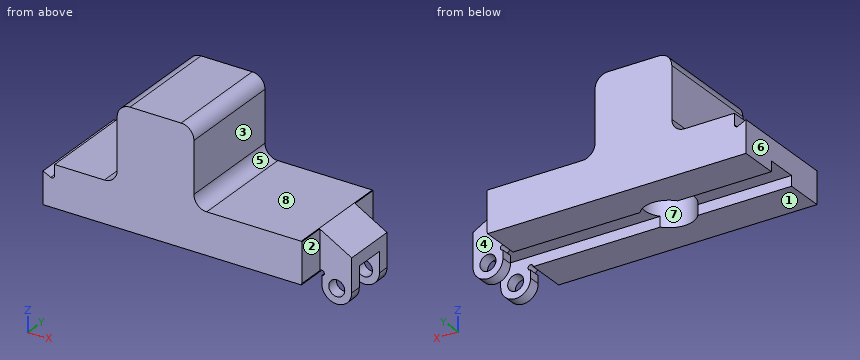
from build123d import *

# Parameters (mm, degrees)
F0_R     = 0.79375
F1_DEPTH = 10.7442
F2_W     = 2.7051
F2_H     = 1.8288
F2_H_2   = 3.302
F2_H_3   = 1.4859
F3_DEPTH = 3.175
F4_R     = 2.413
F5_DEPTH = 11.43
F6_R     = 1.27
F7_R     = 0.254
F8_W     = 3.048
F8_H     = 2.032
F8_H_2   = 1.4859
F9_DEPTH = 28.8808


with BuildPart() as f1:
    # F0 (on Front) → F1 (new body)
    with BuildSketch(Plane.XZ):
        with BuildLine():
            Line((-11.176, 3.175), (-11.176, 0))
            Line((-11.176, 0), (14.478, 0))
            ThreePointArc((14.478, 0), (14.9116051224, 0.1796051224), (14.732, -0.254))
            Line((14.732, -0.254), (14.732, -1.016))
            ThreePointArc((14.732, -1.016), (16.2179, -2.5019), (17.7038, -1.016))
            Line((17.7038, -1.016), (17.7038, 2.286))
            Line((17.7038, 2.286), (14.4678382203, 4.1148))
            Line((14.4678382203, 4.1148), (3.81, 4.1148))
            Line((3.81, 4.1148), (3.81, 11.7348))
            Line((3.81, 11.7348), (-3.81, 11.7348))
            Line((-3.81, 11.7348), (-3.81, 4.1148))
            Line((-3.81, 4.1148), (-10.033, 4.1148))
            Line((-10.033, 4.1148), (-10.033, 2.6214198342))
            Line((-10.033, 2.6214198342), (-11.176, 3.175))
        make_face()
        with Locations((16.2179, -1.016)):
            Circle(F0_R, mode=Mode.SUBTRACT)
    extrude(amount=F1_DEPTH)

    # F2 (on face) → F3 (cut)
    with BuildSketch(Plane.YZ.offset(17.7038)):
        with Locations((-9.39165, 3.2004)):
            Rectangle(F2_W, F2_H)
        with Locations((-9.39165, 0.635)):
            Rectangle(F2_W, F2_H_2)
        with Locations((-9.39165, -1.75895)):
            Rectangle(F2_W, F2_H_3)
        with Locations((-1.35255, 3.2004)):
            Rectangle(F2_W, F2_H)
        with Locations((-1.35255, 0.635)):
            Rectangle(F2_W, F2_H_2)
        with Locations((-1.35255, -1.75895)):
            Rectangle(F2_W, F2_H_3)
    extrude(amount=-F3_DEPTH, mode=Mode.SUBTRACT)

    # F4 (on face) → F5 (cut)
    with BuildSketch(Plane(origin=(0, 0, 0), x_dir=(1, 0, 0), z_dir=(0, 0, -1))):
        with Locations((0, 5.3721)):
            Circle(F4_R)
    extrude(amount=-F5_DEPTH, mode=Mode.SUBTRACT)

    # F6
    f6_edges = [f1.edges().sort_by_distance(p)[0] for p in [
        (-3.81, -5.3721, 4.1148),
        (3.81, -5.3721, 4.1148),
        (-3.81, -5.3721, 11.7348),
        (3.81, -5.3721, 11.7348),
    ]]
    fillet(f6_edges, radius=F6_R)

    # F7
    f7_edges = [f1.edges().sort_by_distance(p)[0] for p in [
        (-10.033, -5.3721, 2.62142),
    ]]
    fillet(f7_edges, radius=F7_R)

    # F8 (on face) → F9 (cut, through all)
    with BuildSketch(Plane.YZ.offset(17.7038)):
        with Locations((-5.3721, 0)):
            Rectangle(F8_W, F8_H)
        with Locations((-5.3721, -1.75895)):
            Rectangle(F8_W, F8_H_2)
    extrude(amount=-F9_DEPTH, mode=Mode.SUBTRACT)


solid = f1.part
Source: CAD feature listing. Evaluate the final solid. Frame: model axes, mm. Face numbers are marked on the shaded views. A direction names the side the tool comes from. Round coordinates to 2 decimals unless told otherwise and drop trailing zeros. Write each loop counter-clockwise with the first axis right and the second up, starting at its lowest first coordinate (ties: lowest second). Pieces come first, ordered by that corner, then holes. Notation, with made-up numbers: M -34.5,85 L 7.5,85 A25 ccw 7.5,110 Z; hole C -10.75,58 d10. An arc over 180 degrees is marked long. One line per item, written item: value. Start each with the question number.
Item 1: Mould query, pull axis X, two halves, no side actions, for the marked faces 5, 6, 7 and 8. Classes: pulls with the +X half, pulls with the -X half, needs draft (parallel to the pull), parting line crosses it, or undercut.
Item 2: Pin query (flat end, axial travel): pin 1 (1.4 mm diameter, centred on x = 16.22, z = -1.02, fed in from -Y); pin 2 (0.8 mm diameter, centred on y = -7.5, z = -0.5, fed in from -X); pin 3 (1.4 mm diameter, centred on y = -1.5, z = 3, fed in from +X); pin 4 (1.5 mm diameter, centred on x = -3, y = -1.5, fed in from -Z). Return the tip coordinate at first contact, or that it passes through.
Item 3: Set-up query: the marked faces 1, 2, 3 and 4. Return all of +Z, -Z, +X, -X, +Y, -Y with unobstructed straight access to the full face (end or side cutting, diameter ignored); none if empty.
Item 4: Ray query, L1, parallel to Z at x = 13.25, y = -2.25; L2, parallel to Y at x = -4, z = 0.75; L3, parallel to Z at x = 2.5, y = -8.5. Return the intervals inside material, ascending. Write a range as from..to.
Item 5: Section query C-C (z = 7). Return the cut outline in (x, y), plus the area to 3 significant figures.
Item 6: Section query A-A (x = 6.5). Return the cut outline in (y, z), plus the area to 3 significant figures.
Item 7: Section query B-B (y = -10). Return the cut outline in (x, z) (3 decimals).
Result set:
1. face 5: pulls with the +X half
1. face 6: pulls with the -X half
1. face 7: undercut
1. face 8: needs draft
2. pin 1: passes through
2. pin 2: stops at x = 14.73
2. pin 3: stops at x = 14.53
2. pin 4: stops at z = 0
3. face 1: -Z, -X, +Y, -Y
3. face 2: +Z, -Z, +X, -Y
3. face 3: +Z, +X, +Y, -Y
3. face 4: +Z, -Z, +X, +Y
4. L1: z = 0..4.11
4. L2: y = -10.74..-6.9, -3.85..0
4. L3: z = 0..11.73
5. outline: M -3.81,-10.74 L 3.81,-10.74 L 3.81,0 L -3.81,0 Z; hole C 0,-5.37 d4.83
5. area: 63.6 mm²
6. outline: M -10.74,0 L -6.9,0 L -6.9,1.02 L -3.85,1.02 L -3.85,0 L 0,0 L 0,4.11 L -10.74,4.11 Z
6. area: 41.1 mm²
7. outline: M -11.176,0 L 14.478,0 A0.254 cw 14.529,0.152 L 14.529,4.08 L 14.468,4.115 L 5.08,4.115 A1.27 cw 3.81,5.385 L 3.81,10.465 A1.27 ccw 2.54,11.735 L -2.54,11.735 A1.27 ccw -3.81,10.465 L -3.81,5.385 A1.27 cw -5.08,4.115 L -10.033,4.115 L -10.033,3.027 A0.254 cw -10.398,2.798 L -11.176,3.175 Z
